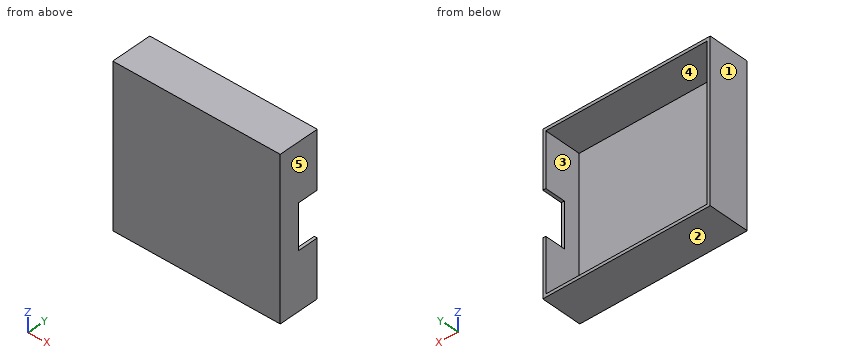
from build123d import *

# Parameters (mm, degrees)
CROQUIS1_W              = 79
CROQUIS1_H              = 75
SALIENTE_EXTRUIR1_DEPTH = 2
SALIENTE_EXTRUIR3_DEPTH = 20
CROQUIS1_5_W            = 1.5
CROQUIS1_5_H            = 22
SALIENTE_EXTRUIR4_DEPTH = 10


with BuildPart() as part:
    # Croquis1 → Saliente-Extruir1 (new body)
    with BuildSketch(Plane(origin=(0, 0, 0), x_dir=(1, 0, 0), z_dir=(0, 1, 0))):
        Rectangle(CROQUIS1_W, CROQUIS1_H)
    extrude(amount=SALIENTE_EXTRUIR1_DEPTH)

    # Croquis1<4> → Saliente-Extruir3 (add)
    with BuildSketch(Plane(origin=(0, 0, 0), x_dir=(1, 0, 0), z_dir=(0, 1, 0))):
        Polygon((-39.5, -37.5), (-39.5, 37.5), (39.5, 37.5), (39.5, 11), (41, 11), (41, 39), (-41, 39), (-41, -39), (41, -39), (41, -11), (39.5, -11), (39.5, -37.5), align=None)
    extrude(amount=SALIENTE_EXTRUIR3_DEPTH)

    # Croquis1<5> → Saliente-Extruir4 (add)
    with BuildSketch(Plane(origin=(0, 0, 0), x_dir=(1, 0, 0), z_dir=(0, 1, 0))):
        with Locations((40.25, 0)):
            Rectangle(CROQUIS1_5_W, CROQUIS1_5_H)
    extrude(amount=SALIENTE_EXTRUIR4_DEPTH)


solid = part.part
Work out the finished part from the listing and answer in its coordinate system (mm). Face numbers are marked on the shaded views. A direction names the side the tool comes from. Coordinates: 2 decimals unless noted, no trailing zeros. Write each loop counter-clockwise with the first axis right and the second up, starting at its lowest first coordinate (ties: lowest second). Pieces come first, ordered by that corner, then holes. Notation, with made-up numbers: M -13.75,14 L 26.25,14 A11 cw 26.25,24 Z; hole C 70,-38 d2. An arc over 180 degrees is marked long. Use one line per item in the form item = value. Start each with the question number.
1. The part is cut by section C-C (x = 10.5). Give the vertices of the cut face in (y, z).
2. The mould has two halves that part along X. Classify the marked faces 1, 2 and 3: released by +X, released by -X, zero draft, split by the parting line, or undercut.
3. The part is cut by section B-B (z = -10). Give the vertices of the cut face in (x, y), plus the area to 3 significant figures.
4. A tool of negligible diameter and unlimited length cuts with its end or side. For the marked faces 4 and 5, from which of +Z, -Z, +X, -X, +Y, -Y can it reach the whole face along a straight path? Write none if from no direction.
5. Straight lines are drawn through the part: probe 1 along Z at (x, y) = (10.5, 12); probe 2 along X at (y, z) = (17, 30.5); probe 3 along Y at (x, z) = (-30, 7). For each, find the intervals that lie inside material, in ascending order. Write a range as from..to.
6. Each of these flat-tipped pins is pushed along its axis until it touches: P1, Ø1, axis at x = 27.5, z = -23, coming from the -Y side; P2, Ø8, axis at x = -2, z = 12, coming from the +Y side; P3, Ø0.8, axis at x = 40.5, z = 0.5, coming from the +Y side. Where does it stop, or does it pass through?
7. The part is cut by section A-A (y = 18). Give the vertices of the cut face in (x, z), plus the area to 3 significant figures.
8. The part is cut by section D-D (y = 8.5). Give the vertices of the cut face in (x, z), plus the area to 3 significant figures.
Evaluation:
q1.outline = M 0,-39 L 20,-39 L 20,-37.5 L 2,-37.5 L 2,37.5 L 20,37.5 L 20,39 L 0,39 Z
q2.face_1 = released by -X
q2.face_2 = zero draft
q2.face_3 = undercut
q3.outline = M -41,0 L 41,0 L 41,10 L 39.5,10 L 39.5,2 L -39.5,2 L -39.5,20 L -41,20 Z
q3.area = 203 mm^2
q4.face_4 = +Y
q4.face_5 = +Z, -Z, +X, +Y, -Y
q5.probe_1 = -39..-37.5, 37.5..39
q5.probe_2 = -41..-39.5, 39.5..41
q5.probe_3 = 0..2
q6.P1 = 0
q6.P2 = 2
q6.P3 = 10
q7.outline = M -41,-39 L 41,-39 L 41,-11 L 39.5,-11 L 39.5,-37.5 L -39.5,-37.5 L -39.5,37.5 L 39.5,37.5 L 39.5,11 L 41,11 L 41,39 L -41,39 Z
q7.area = 438 mm^2
q8.outline = M -41,-39 L 41,-39 L 41,39 L -41,39 Z; hole M -39.5,-37.5 L 39.5,-37.5 L 39.5,37.5 L -39.5,37.5 Z
q8.area = 471 mm^2
